from build123d import *

# Parameters (mm, degrees)
SKETCH1_W            = 60
SKETCH1_H            = 60
BOSS_EXTRUDE1_DEPTH  = 9.525
M5_CLEARANCE_HOLE1_D = 5.3
SKETCH5_R            = 8
CUT_EXTRUDE1_DEPTH   = 4.572
SKETCH6_R            = 6.35
CUT_EXTRUDE2_DEPTH   = 5.953


with BuildPart() as part:
    # Sketch1 → Boss-Extrude1 (new body)
    with BuildSketch(Plane(origin=(0, 0, 0), x_dir=(1, 0, 0), z_dir=(0, 1, 0))):
        Rectangle(SKETCH1_W, SKETCH1_H)
    extrude(amount=BOSS_EXTRUDE1_DEPTH)

    # M5 Clearance Hole1 (through all)
    with Locations(Plane(origin=(0, 9.525, 0), x_dir=(1, 0, 0), z_dir=(0, 1, 0))):
        with Locations((-23.57, 23.57), (23.57, 23.57), (23.57, -23.57), (-23.57, -23.57)):
            Hole(M5_CLEARANCE_HOLE1_D / 2)

    # Sketch5 → Cut-Extrude1 (cut)
    with BuildSketch(Plane(origin=(0, 9.525, 0), x_dir=(1, 0, 0), z_dir=(0, 1, 0))):
        Circle(SKETCH5_R)
    extrude(amount=-CUT_EXTRUDE1_DEPTH, mode=Mode.SUBTRACT)

    # Sketch6 → Cut-Extrude2 (cut, through all)
    with BuildSketch(Plane(origin=(0, 4.953, 0), x_dir=(1, 0, 0), z_dir=(0, 1, 0))):
        Circle(SKETCH6_R)
    extrude(amount=-CUT_EXTRUDE2_DEPTH, mode=Mode.SUBTRACT)


solid = part.part
Work out the finished part from the listing and answer in its coordinate system (mm). A direction names the side the tool comes from. Round coordinates to 2 decimals unless told otherwise and drop trailing zeros. Order: outer loops, then holes, each group sorted by start corner. A loop starts at its lowest first (then second) coordinate and runs counter-clockwise, first axis right, second up. Notation, with made-up numbers: M 33,68 L 91,68 A17 ccw 91,80 Z; hole C -27,-23.75 d11. An arc over 180 degrees is marked long. Put each result on its own line as item: value. Start each with the question number.
Q1. For a pull along Z with two mould halves and no side action, classify faces 1 (the cylindrical face through (22.145, 4.696, -25.804)), 2 (the cylindrical face through (-1.38, 2.51, 6.2)), 3 (the flat face through (0, 5, -30)), 4 (the flat face through (-30, 5, 0)) as pulls with the +Z half, pulls with the -Z half, needs draft (parallel to the pull), parting line crosses it, or undercut.
Q2. Section B-B, the plane x = 23.57 is taken. Write down the section's boundary in (y, z) (3 decimals).
Q3. Straight lines are drawn through the part: L1, parallel to Z at x = -23.57, y = 2.5; L2, parallel to Z at x = 22.5, y = 9. For each, find the intervals that lie inside material, in ascending order. Write a range as [from, to].
Q4. Section C-C, the plane z = 0 is taken. Write down the section's boundary in (x, y) (3 decimals).
Q5. A tool of negligible diameter and unlimited length cuts with its end or side. For faces 5 (the flat face through (0, 5, 30)), 6 (the cylindrical face through (-1.73, 7.27, 7.81)), from which of +Z, -Z, +X, -X, +Y, -Y can it reach the whole face along a straight path? Write none if from no direction.
Q6. Flat-ended cylindrical pins translate along their axes: pin 1 (9.5 mm diameter, centred on x = 0, z = 0, fed in from -Y); pin 2 (10 mm diameter, centred on x = -15, z = -19.5, fed in from -Y); pin 3 (8 mm diameter, centred on x = 2, z = 1.5, fed in from +Y). Find the tip coordinate at first contact, or state that the pin passes through.
Q7. Section D-D, the plane x = 0 is taken. Write down the section's boundary in (y, z) (3 decimals).
Q8. Section A-A, the plane z = 23.57 is taken. Write down the section's boundary in (x, y) (3 decimals).
Findings below:
1. face 1: undercut
1. face 2: undercut
1. face 3: pulls with the -Z half
1. face 4: needs draft
2. outline: M 0,-30 L 9.525,-30 L 9.525,-26.22 L 0,-26.22 Z; M 0,-20.92 L 9.525,-20.92 L 9.525,20.92 L 0,20.92 Z; M 0,26.22 L 9.525,26.22 L 9.525,30 L 0,30 Z
3. L1: z = [-30, -26.22], [-20.92, 20.92], [26.22, 30]
3. L2: z = [-30, -25.99], [-21.15, 21.15], [25.99, 30]
4. outline: M -30,0 L -6.35,0 L -6.35,4.953 L -8,4.953 L -8,9.525 L -30,9.525 Z; M 6.35,0 L 30,0 L 30,9.525 L 8,9.525 L 8,4.953 L 6.35,4.953 Z
5. face 5: +Z, +X, -X, +Y, -Y
5. face 6: +Y
6. pin 1: passes through
6. pin 2: stops at y = 0
6. pin 3: stops at y = 4.95
7. outline: M 0,-30 L 9.525,-30 L 9.525,-8 L 4.953,-8 L 4.953,-6.35 L 0,-6.35 Z; M 0,6.35 L 4.953,6.35 L 4.953,8 L 9.525,8 L 9.525,30 L 0,30 Z
8. outline: M -30,0 L -26.22,0 L -26.22,9.525 L -30,9.525 Z; M -20.92,0 L 20.92,0 L 20.92,9.525 L -20.92,9.525 Z; M 26.22,0 L 30,0 L 30,9.525 L 26.22,9.525 Z
